The model under review builds one solid part; all positions refer to its coordinate system, in mm. A direction names the side the tool comes from. Give positions to 0.01 mm unless a question says otherwise; leave off trailing zeros. Write each loop counter-clockwise with the first axis right and the second up, starting at its lowest first coordinate (ties: lowest second). Pieces come first, ordered by that corner, then holes. Notation, with made-up numbers: (22.25, 82.5) - (40.25, 82.5) arc R9 cw to (40.25, 91.5) - close; hole circle Ø3 at (48.25, 65.25). An arc over 180 degrees is marked (long way). One line per question, with ' | ' between items. Start each with the question number.
```python
from build123d import *

# Parameters (mm, degrees)
SKETCH1_R           = 5.08
BOSS_EXTRUDE1_DEPTH = 2.9972


with BuildPart() as part:
    # Sketch1 → Boss-Extrude1 (new body)
    with BuildSketch(Plane(origin=(0, 0, 0), x_dir=(1, 0, 0), z_dir=(0, 1, 0))):
        Circle(SKETCH1_R)
        with BuildLine():
            Line((-1.9685, 1.4605), (1.9685, 1.4605))
            ThreePointArc((1.9685, 1.4605), (2.451132901, 0), (1.9685, -1.4605))
            Line((1.9685, -1.4605), (-1.9685, -1.4605))
            ThreePointArc((-1.9685, -1.4605), (-2.451132901, 0), (-1.9685, 1.4605))
        make_face(mode=Mode.SUBTRACT)
    extrude(amount=BOSS_EXTRUDE1_DEPTH)


solid = part.part
```
Item 1: Take a section at D-D (z = 4.75). Give the boundary of the cut face in (x, y).
Item 2: The part is to be moulded in two halves that separate along X. For faces 1 (the flat face through (0, 2.997, 2)), 2 (the cylindrical face through (-2.45, 1.48, 0.02)), 3 (the flat face through (0, 1, -1.46)), 4 (the cylindrical face through (-0.661, 1.478, -5.037)), say which applies: +X half, -X half, draft (parallel to the pull), parting line (faces both ways), or undercut.
Item 3: For probe 1 along Z at (x, y) = (2.25, 1); probe 2 along X at (y, z) = (1.15, -0.25); probe 3 along Z at (x, y) = (-1, 0.7), list the stretches that pass through material, from the lowest coordinate up.
Item 4: Take a section at B-B (x = 0). Give the boundary of the cut face in (y, z).
Item 5: Clearance check with flat-ended pins moving along their axes: P1, Ø1.5, axis at x = 2.5, y = 0.5, coming from the -Z side; P2, Ø1.5, axis at y = 0.5, z = -2.5, coming from the -X side. State where each tip first meets the part, or that it passes through.
Item 6: Machinability: for faces 5 (the flat face through (0, 0, 2)), 6 (the flat face through (0, 1, 1.46)), which of the approach directions +Z, -Z, +X, -X, +Y, -Y give a long, thin tool a straight path to every point of the face, cutting with its end or side? Answer none if there is none.
Item 7: Take a section at A-A (z = 0). Give the boundary of the cut face in (x, y), plus the area to 3 significant figures.
Item 8: Take a section at C-C (y = 2). Give the boundary of the cut face in (x, z).
Check sheet entries:
1) outline: (-1.8, 0) - (1.8, 0) - (1.8, 3) - (-1.8, 3) - close
2) face 1: draft | face 2: undercut | face 3: undercut | face 4: parting line
3) probe 1: z = -4.55 to -0.97, 0.97 to 4.55 | probe 2: x = -5.07 to -2.44, 2.44 to 5.07 | probe 3: z = -4.98 to -1.46, 1.46 to 4.98
4) outline: (0, -5.08) - (3, -5.08) - (3, -1.46) - (0, -1.46) - close; (0, 1.46) - (3, 1.46) - (3, 5.08) - (0, 5.08) - close
5) P1: stops at z = -4.77 | P2: stops at x = -4.77
6) face 5: +Z, -Z, +X, -X, -Y | face 6: +Y, -Y
7) outline: (-5.08, 0) - (-2.45, 0) - (-2.45, 3) - (-5.08, 3) - close; (2.45, 0) - (5.08, 0) - (5.08, 3) - (2.45, 3) - close | area: 15.8 mm^2
8) outline: circle Ø10.16 at (0, 0); hole (-1.97, -1.46) - (1.97, -1.46) arc R2.45 ccw to (1.97, 1.46) - (-1.97, 1.46) arc R2.45 ccw to start
